Print and shaded views of the part. All mm, measured from the part's lowest x, y and z. A direction names the side the tool comes from. Coordinates: 2 decimals unless noted, no trailing zeros. Order: outer loops, then holes, each group sorted by start corner. A loop starts at its lowest first (then second) coordinate and runs counter-clockwise, first axis right, second up. Notation, with made-up numbers: (2, 66.25) -> (30, 66.25) arc R8 cw to (30, 73.25) -> close; hole circle Ø11 at (78, 5). An arc over 180 degrees is marked (long way). Return JSON: item names as keys, results as strings. Group by question number.
1) Cut at C-C (y = 15.25). Write the cut outline in (x, z).
2) Flat gauge pins, fed straight in: pin 1 (2 mm diameter, centred on x = 19.5, z = 5, fed in from +Y); pin 2 (6 mm diameter, centred on x = 26, z = 12, fed in from +Y). Where does each tip first touch, or does it go through?
3) Which spindle directions (+Z, -Z, +X, -X, +Y, -Y) get a long thin tool onto all of the face, cutting with end or side? Do the marked faces 4 and 5. Say none if no direction does.
4) Cut at A-A (z = 12). Write the cut outline in (x, y), and give its area (3 significant figures).
5) Pull direction Z, two halves, no side cores. Call the marked faces 1, 2 and 3: +Z half, -Z half, draft (parallel to the pull), parting line (faces both ways), or undercut.
6) Cut at D-D (z = 3.5). Write the cut outline in (x, y).
7) Cut at B-B (x = 26). Write the cut outline in (y, z), and give its area (3 significant figures).
8) Probe line 1 (Z direction, x = 26, y = 21.2); line 2 (X direction, y = 21.3, z = 12); line 3 (Y direction, x = 5, z = 13). List the from-to ranges inside material, lowest first.
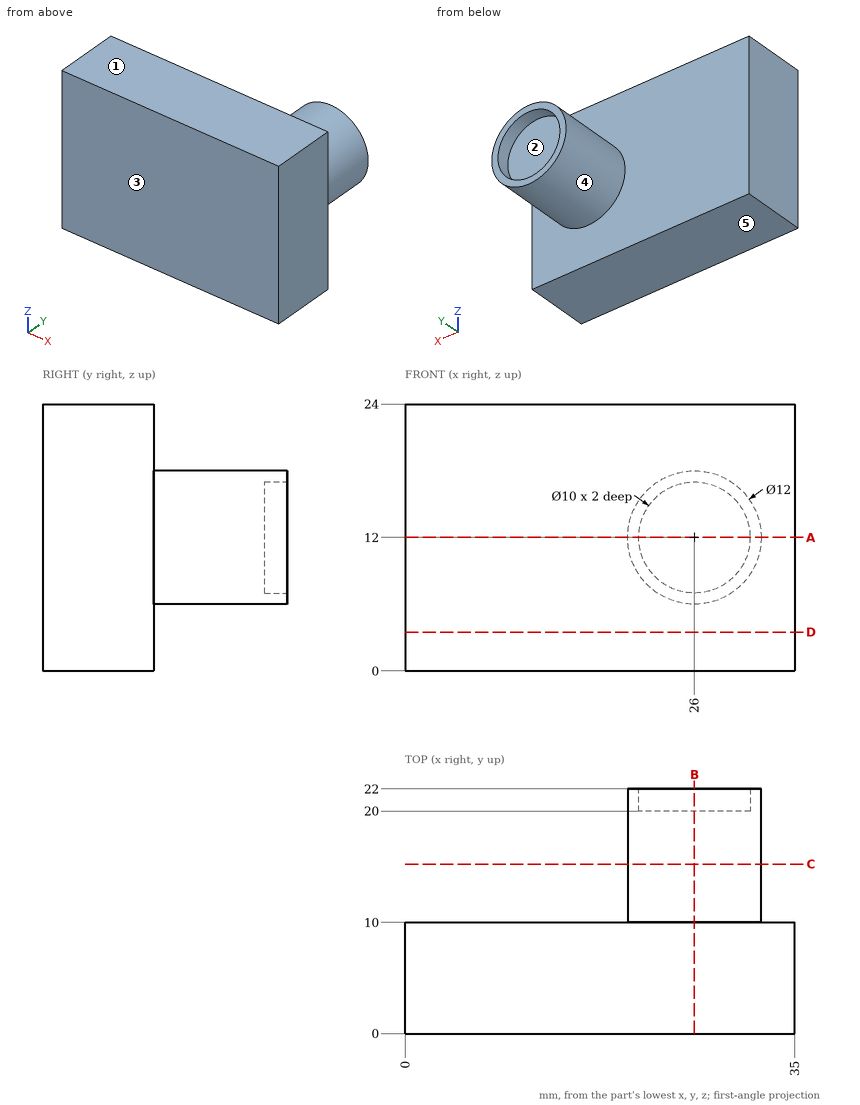
Answers below:
{
 "1": {"outline": "circle Ø12 at (26, 12)"},
 "2": {"pin 1": "stops at y = 10", "pin 2": "stops at y = 20"},
 "3": {"face 4": "+Y", "face 5": "-Z, +X, -X, +Y, -Y"},
 "4": {"outline": "(0, 0) -> (35, 0) -> (35, 10) -> (32, 10) -> (32, 22) -> (31, 22) -> (31, 20) -> (21, 20) -> (21, 22) -> (20, 22) -> (20, 10) -> (0, 10) -> close", "area": "474 mm^2"},
 "5": {"face 1": "+Z half", "face 2": "undercut", "face 3": "draft"},
 "6": {"outline": "(0, 0) -> (35, 0) -> (35, 10) -> (0, 10) -> close"},
 "7": {"outline": "(0, 0) -> (10, 0) -> (10, 6) -> (22, 6) -> (22, 7) -> (20, 7) -> (20, 17) -> (22, 17) -> (22, 18) -> (10, 18) -> (10, 24) -> (0, 24) -> close", "area": "364 mm^2"},
 "8": {"line 1": "z = 6 to 7, 17 to 18", "line 2": "x = 20 to 21, 31 to 32", "line 3": "y = 0 to 10"}
}
